Read the model definition and answer for the solid it produces. Units are mm, in the model's axes. Face numbers are marked on the shaded views. A direction names the side the tool comes from. Round coordinates to 2 decimals unless told otherwise and drop trailing zeros. Loops run counter-clockwise (first coordinate to the right, second up) from the corner with the lowest first, then second, coordinate; pieces in that order, holes last. Notation, with made-up numbers: M 52.5,41 L 106.5,41 A31 cw 106.5,74 Z; hole C 71.25,-16.75 d3. An arc over 180 degrees is marked long. Write each question's results on one line, items separated by ' | '.
from build123d import *

# Parameters (mm, degrees)
F0_W      = 42.3
F0_H      = 42.3
F1_DEPTH  = 59
F2_R      = 11
F3_DEPTH  = 2
F4_R      = 2.5
F5_DEPTH  = 22
F7_DEPTH  = 15
F9_DEPTH  = 4.5
F10_DEPTH = 61


with BuildPart() as f1:
    # F0 (on Front) → F1 (new body)
    with BuildSketch(Plane.XZ):
        Rectangle(F0_W, F0_H)
    extrude(amount=F1_DEPTH)

    # F2 (on face) → F3 (join)
    with BuildSketch(Plane.XZ.offset(59)):
        Circle(F2_R)
    extrude(amount=F3_DEPTH)

    # F4 (on face) → F5 (join)
    with BuildSketch(Plane.XZ.offset(61)):
        Circle(F4_R)
    extrude(amount=F5_DEPTH)

    # F6 (on face) → F7 (cut)
    with BuildSketch(Plane.XZ.offset(83)):
        with BuildLine():
            ThreePointArc((0, 2.5), (-0.790569415, 2.3717082451), (-1.5, 2))
            Line((-1.5, 2), (0, 2))
            Line((0, 2), (0, 2.5))
        make_face()
        with BuildLine():
            Line((0, 2.5), (0, 2))
            Line((0, 2), (1.5, 2))
            ThreePointArc((1.5, 2), (0.790569415, 2.3717082451), (0, 2.5))
        make_face()
    extrude(amount=-F7_DEPTH, mode=Mode.SUBTRACT)

    # F8 (on face) → F9 (cut)
    with BuildSketch(Plane.XZ.offset(59)):
        with BuildLine():
            ThreePointArc((16.75, 15.5), (15.5, 16.75), (14.25, 15.5))
            Line((14.25, 15.5), (15.5, 15.5))
            Line((15.5, 15.5), (15.5, 14.25))
            ThreePointArc((15.5, 14.25), (16.3838834765, 14.6161165235), (16.75, 15.5))
        make_face()
        with BuildLine():
            Line((15.5, 15.5), (14.25, 15.5))
            ThreePointArc((14.25, 15.5), (14.6161165235, 14.6161165235), (15.5, 14.25))
            Line((15.5, 14.25), (15.5, 15.5))
        make_face()
        with BuildLine():
            Line((-15.5, 14.25), (-15.5, 15.5))
            Line((-15.5, 15.5), (-14.25, 15.5))
            ThreePointArc((-14.25, 15.5), (-16.3838834765, 16.3838834765), (-15.5, 14.25))
        make_face()
        with BuildLine():
            Line((-14.25, 15.5), (-15.5, 15.5))
            Line((-15.5, 15.5), (-15.5, 14.25))
            ThreePointArc((-15.5, 14.25), (-14.6161165235, 14.6161165235), (-14.25, 15.5))
        make_face()
        with BuildLine():
            Line((-15.5, -15.5), (-15.5, -14.25))
            ThreePointArc((-15.5, -14.25), (-16.3838834765, -16.3838834765), (-14.25, -15.5))
            Line((-14.25, -15.5), (-15.5, -15.5))
        make_face()
        with BuildLine():
            ThreePointArc((-14.25, -15.5), (-14.6161165235, -14.6161165235), (-15.5, -14.25))
            Line((-15.5, -14.25), (-15.5, -15.5))
            Line((-15.5, -15.5), (-14.25, -15.5))
        make_face()
        with BuildLine():
            Line((15.5, -15.5), (15.5, -14.25))
            ThreePointArc((15.5, -14.25), (14.6161165235, -14.6161165235), (14.25, -15.5))
            Line((14.25, -15.5), (15.5, -15.5))
        make_face()
        with BuildLine():
            ThreePointArc((16.75, -15.5), (16.3838834765, -14.6161165235), (15.5, -14.25))
            Line((15.5, -14.25), (15.5, -15.5))
            Line((15.5, -15.5), (14.25, -15.5))
            ThreePointArc((14.25, -15.5), (15.5, -16.75), (16.75, -15.5))
        make_face()
    extrude(amount=-F9_DEPTH, mode=Mode.SUBTRACT)

    # F10 (cut): a face of the model
    f10_faces = [f1.faces().sort_by_distance(p)[0] for p in [
        (0, 0, 0),
    ]]
    extrude(f10_faces, amount=-F10_DEPTH, mode=Mode.SUBTRACT)


solid = f1.part
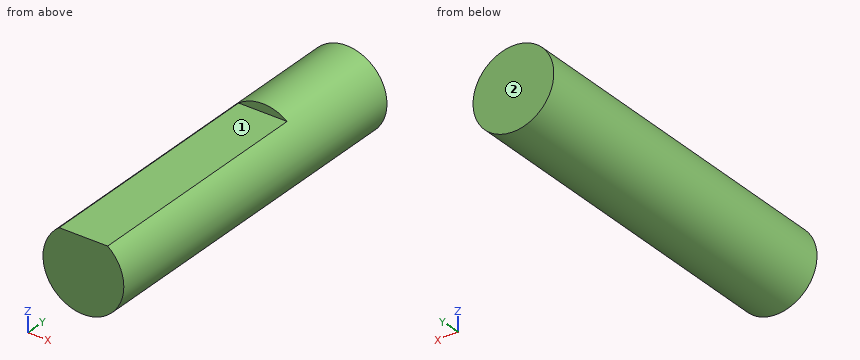
Item 1: The part is cut by section A-A (x = 0). Determine the outline of the cut face in (y, z).
Outcome:
outline: M -83,-2.5 L -61,-2.5 L -61,2.5 L -68,2.5 L -68,2 L -83,2 Z
Item 2: Straight lines are drawn through the part: line 1 (Z direction, x = -0.1, y = -72.75); line 2 (Z direction, x = 2, y = -67); line 3 (X direction, y = -75.5, z = -1.65). For each, find the intervals that lie inside material, in ascending order.
Outcome:
line 1: z = -2.5 to 2 | line 2: z = -1.5 to 1.5 | line 3: x = -1.88 to 1.88
Item 3: The part is cut by section B-B (y = -72). Determine the outline of the cut face in (x, z).
Outcome:
outline: M -1.5,2 A2.5 ccw long 1.5,2 Z
Item 4: For the marked faces 1 and 2, determine the directions among +Z, -Z, +X, -X, +Y, -Y from which every point of the face is accessible in a straight line to the end or side of a thin tool.
Outcome:
face 1: +Z, +X, -X, -Y | face 2: +Z, -Z, +X, -X, +Y
Item 5: The part is cut by section D-D (x = 1.05). Determine the outline of the cut face in (y, z).
Outcome:
outline: M -83,-2.27 L -61,-2.27 L -61,2.27 L -68,2.27 L -68,2 L -83,2 Z
Item 6: The part is cut by section C-C (z = -0.6). Determine the outline of the cut face in (x, y), plus the area to 3 significant figures.
Outcome:
outline: M -2.43,-83 L 2.43,-83 L 2.43,-61 L -2.43,-61 Z | area: 107 mm2
